```python
from build123d import *

# Parameters (mm, degrees)
BOSS_EXTRUDE1_DEPTH             = 3.5
CUT_EXTRUDE1_REACH              = 24.897
SKETCH2_R                       = 1.6
FILLET1_R                       = 1.5
FILLET1_OF_MIRROR1_R            = 1.5
SKETCH3_R                       = 9.5
SKETCH3_R_2                     = 8
BOSS_EXTRUDE3_DEPTH             = 15
BOSS_EXTRUDE3_DIRECTION_2_REACH = 25.953


with BuildPart() as part:
    # Sketch1 → Boss-Extrude1 (new body)
    with BuildSketch(Plane(origin=(0, 0, 0), x_dir=(1, 0, 0), z_dir=(0, 1, 0))):
        Polygon((-12, 0), (-12, 7.5), (-16, 11), (-16, 16), (16, 16), (16, 11), (12, 7.5), (12, 0), align=None)
    boss_extrude1 = extrude(amount=BOSS_EXTRUDE1_DEPTH)

    # Sketch2 → Cut-Extrude1 (cut, up to next)
    with BuildSketch(Plane(origin=(0, 3.5, 0), x_dir=(1, 0, 0), z_dir=(0, 1, 0)), mode=Mode.PRIVATE) as cut_extrude1_sk1:
        with Locations(Location((-12.5, 13.5, 0), (0, 0, 270))):
            Circle(SKETCH2_R)
    cut_extrude1_tool1 = extrude(cut_extrude1_sk1.sketch, amount=-CUT_EXTRUDE1_REACH, mode=Mode.PRIVATE) & part.part
    # Sketch2 → Cut-Extrude1 (cut, up to next)
    with BuildSketch(Plane(origin=(0, 3.5, 0), x_dir=(1, 0, 0), z_dir=(0, 1, 0)), mode=Mode.PRIVATE) as cut_extrude1_sk2:
        with Locations(Location((12.5, 13.5, 0), (0, 0, 270))):
            Circle(SKETCH2_R)
    cut_extrude1_tool2 = extrude(cut_extrude1_sk2.sketch, amount=-CUT_EXTRUDE1_REACH, mode=Mode.PRIVATE) & part.part
    cut_extrude1_1 = cut_extrude1_tool1.solids().sort_by_distance((-12.5, 3.5, -13.5))[0]
    add(cut_extrude1_1, mode=Mode.SUBTRACT)
    cut_extrude1_2 = cut_extrude1_tool2.solids().sort_by_distance((12.5, 3.5, -13.5))[0]
    add(cut_extrude1_2, mode=Mode.SUBTRACT)
    cut_extrude1 = cut_extrude1_1 + cut_extrude1_2  # Cut-Extrude1 as one shape, for the pattern or mirror that repeats it

    # Fillet1
    fillet1_edges = [part.edges().sort_by_distance(p)[0] for p in [
        (-12, 1.75, -7.5),
        (-16, 1.75, -11),
        (-16, 1.75, -16),
        (16, 1.75, -16),
        (16, 1.75, -11),
        (12, 1.75, -7.5),
    ]]
    fillet(fillet1_edges, radius=FILLET1_R)

    # Mirror1: Boss-Extrude1, Cut-Extrude1 across plane
    add(boss_extrude1.mirror(Plane.XY))
    add(cut_extrude1.mirror(Plane.XY), mode=Mode.SUBTRACT)

    # Fillet1 of Mirror1
    fillet1_of_mirror1_edges = [part.edges().sort_by_distance(p)[0] for p in [
        (-12, 1.75, 7.5),
        (-16, 1.75, 11),
        (-16, 1.75, 16),
        (16, 1.75, 16),
        (16, 1.75, 11),
        (12, 1.75, 7.5),
    ]]
    fillet(fillet1_of_mirror1_edges, radius=FILLET1_OF_MIRROR1_R)

    # Sketch3 → Boss-Extrude3 (add)
    with BuildSketch(Plane(origin=(-1.403733341, 3.856725658, 0), x_dir=(0, 0, 1), z_dir=(-0.34202014332566977, 0.939692620785908, 0))):
        with Locations(Location((0, 1.197070502, 0), (0, 0, 270))):
            Circle(SKETCH3_R)
        with Locations(Location((0, 1.197070502, 0), (0, 0, 270))):
            Circle(SKETCH3_R_2, mode=Mode.SUBTRACT)
    extrude(amount=BOSS_EXTRUDE3_DEPTH)

    # Boss-Extrude3 direction 2: up to this face of the body (flat: up to its plane)
    boss_extrude3_direction_2_end = Plane(part.part.faces().sort_by_distance((0, 3.5, 0))[0])
    # Sketch3 → Boss-Extrude3 direction 2 (add, up to the picked face)
    with BuildSketch(Plane(origin=(-1.403733341, 3.856725658, 0), x_dir=(0, 0, 1), z_dir=(-0.34202014332566977, 0.939692620785908, 0)), mode=Mode.PRIVATE) as boss_extrude3_direction_2_sk1:
        with Locations(Location((0, 1.197070502, 0), (0, 0, 270))):
            Circle(SKETCH3_R)
        with Locations(Location((0, 1.197070502, 0), (0, 0, 270))):
            Circle(SKETCH3_R_2, mode=Mode.SUBTRACT)
    boss_extrude3_direction_2_tool1 = split(extrude(boss_extrude3_direction_2_sk1.sketch, amount=-BOSS_EXTRUDE3_DIRECTION_2_REACH, mode=Mode.PRIVATE), bisect_by=boss_extrude3_direction_2_end, keep=Keep.BOTH, mode=Mode.PRIVATE)
    add(boss_extrude3_direction_2_tool1.solids().sort_by(Axis((8.395729, 7.423438, 0), (0.34202014332566977, -0.939692620785908, 0)))[0])


solid = part.part
```
Check sheet for the modelled part. Datum: model origin and axes. Units: mm. A direction names the side the tool comes from. Coordinates: 2 decimals unless noted, no trailing zeros. Write each loop counter-clockwise with the first axis right and the second up, starting at its lowest first coordinate (ties: lowest second). Pieces come first, ordered by that corner, then holes. Notation, with made-up numbers: (20, 2.5) -> (55, 2.5) arc R33 cw to (55, 34.5) -> close; hole circle Ø7 at (36, 47.5). An arc over 180 degrees is marked (long way). Use a Markdown table: item, result.
1. Sectioned sample at C-C (z = -14). Enter the section's corners in (x, y).
Reported:
| item | result |
|---|---|
| outline | (-16, 0) -> (-14.02, 0) -> (-14.02, 3.5) -> (-16, 3.5) -> close; (-10.98, 0) -> (10.98, 0) -> (10.98, 3.5) -> (-10.98, 3.5) -> close; (14.02, 0) -> (16, 0) -> (16, 3.5) -> (14.02, 3.5) -> close |
2. Release check for a two-part mould opening along Z. For faces 1 (the cylindrical face through (-15.57, 1.77, -15.55)), 2 (the flat face through (14.02, 1.73, 9.27)), 3 (the flat face through (16, 2, -13)) record: pulls with the +Z half, pulls with the -Z half, needs draft (parallel to the pull), parting line crosses it, or undercut.
Reported:
| item | result |
|---|---|
| face 1 | pulls with the -Z half |
| face 2 | undercut |
| face 3 | needs draft |
3. Go/stop test with flat-tipped pins: pin 1 Ø2 at (x, z) = (10.5, 11) entering from +Y; pin 2 Ø3 at (y, z) = (2, -1.5) entering from -X; pin 3 Ø6 at (x, z) = (5.5, 8) entering from -Y; pin 4 Ø16 at (x, z) = (-4.5, 1.5) entering from +Y. Record where each tip stops, or that it passes through.
Reported:
| item | result |
|---|---|
| pin 1 | stops at y = 3.5 |
| pin 2 | stops at x = -12 |
| pin 3 | stops at y = 0 |
| pin 4 | stops at y = 21.6 |
4. Scan lines: line 1 along X through (y, z) = (1, 13.5); line 2 along Y through (x, z) = (-10.5, 8); line 3 along X through (y, z) = (5, -7). Record each from-to range of solid material in increasing order.
Reported:
| item | result |
|---|---|
| line 1 | x = -16 to -14.1, -10.9 to 10.9, 14.1 to 16 |
| line 2 | y = 0 to 3.5 |
| line 3 | x = -7.38 to -4.67, 3.58 to 6.29 |
5. Tool access check on faces 4 (the flat face through (-12, 2, 0)), 5 (the flat face through (0, 0, 0)), 6 (the flat face through (14.02, 1.73, -9.27)), 7 (the cylindrical face through (-12.43, 1.77, 15.1)), 8 (the flat face through (-13.98, 1.73, 9.23)). Record the directions out of +Z, -Z, +X, -X, +Y, -Y that give a thin tool (end or side, any length) a straight path to the whole face; none if there is none.
Reported:
| item | result |
|---|---|
| face 4 | -X, -Y |
| face 5 | +Z, -Z, +X, -X, -Y |
| face 6 | +X, +Y, -Y |
| face 7 | +Y, -Y |
| face 8 | -X, +Y, -Y |
6. Sectioned sample at B-B (z = -5.5). Enter the section's corners in (x, y), plus the area to 3 significant figures.
Reported:
| item | result |
|---|---|
| outline | (-12.69, 15.71) -> (-8.24, 3.5) -> (-12, 3.5) -> (-12, 0) -> (12, 0) -> (12, 3.5) -> (8.24, 3.5) -> (1.87, 21.01) -> (0.05, 20.35) -> (6.18, 3.5) -> (-6.18, 3.5) -> (-10.87, 16.37) -> close |
| area | 145 mm2 |
7. Sectioned sample at A-A (z = 13.5). Enter the section's corners in (x, y).
Reported:
| item | result |
|---|---|
| outline | (-16, 0) -> (-14.1, 0) -> (-14.1, 3.5) -> (-16, 3.5) -> close; (-10.9, 0) -> (10.9, 0) -> (10.9, 3.5) -> (-10.9, 3.5) -> close; (14.1, 0) -> (16, 0) -> (16, 3.5) -> (14.1, 3.5) -> close |
8. Sectioned sample at D-D (z = 1). Enter the section's corners in (x, y).
Reported:
| item | result |
|---|---|
| outline | (-14.29, 15.13) -> (-10.05, 3.5) -> (-12, 3.5) -> (-12, 0) -> (12, 0) -> (12, 3.5) -> (10.05, 3.5) -> (3.47, 21.59) -> (2.05, 21.08) -> (8.45, 3.5) -> (-8.45, 3.5) -> (-12.87, 15.65) -> close |
